from build123d import *

# Parameters (mm, degrees)
SKETCH1_R               = 114.3
BOSS_EXTRUDE1_DEPTH     = 762
SKETCH2_R               = 76.2
CUT_EXTRUDE1_DEPTH      = 94.996
CUT_EXTRUDE2_DEPTH      = 241.046
CUT_EXTRUDE2_DEPTH_BACK = 276.352
SKETCH6_R               = 150.368


with BuildPart() as part:
    # Sketch1 → Boss-Extrude1 (new body)
    with BuildSketch(Plane.XY):
        Circle(SKETCH1_R)
    extrude(amount=BOSS_EXTRUDE1_DEPTH)

    # Sketch2 → Cut-Extrude1 (cut)
    with BuildSketch(Plane.XY.offset(762)):
        Circle(SKETCH2_R)
    extrude(amount=-CUT_EXTRUDE1_DEPTH, mode=Mode.SUBTRACT)

    # Sketch6 → Cut-Extrude2 (cut, two sides: drawn at the far end of the back side and taken through both)
    with BuildSketch(Plane(origin=(0, 0, 0), x_dir=(1, 0, 0), z_dir=(0, 1, 0)).offset(-CUT_EXTRUDE2_DEPTH_BACK)):
        Circle(SKETCH6_R)
    extrude(amount=CUT_EXTRUDE2_DEPTH + CUT_EXTRUDE2_DEPTH_BACK, mode=Mode.SUBTRACT)


solid = part.part
Part model, mm, in its own coordinate system. A direction names the side the tool comes from. Give positions to 0.01 mm unless a question says otherwise; leave off trailing zeros. Loops run counter-clockwise (first coordinate to the right, second up) from the corner with the lowest first, then second, coordinate; pieces in that order, holes last. Notation, with made-up numbers: M -14,-38.75 L 6,-38.75 A11 ccw 6,-19.75 Z; hole C -35.75,89 d1. An arc over 180 degrees is marked long. Put each result on its own line as item: value. Start each with the question number.
1) Saw through at A-A (y = 0). List the corners of the cut face in (x, z), then the cut area to 3 significant figures.
2) Pull direction Y, two halves, no side cores. Call faces 1 (the flat face through (-1, 1, 667.004)), 2 (the cylindrical face through (-114.19, 5.03, 425.2)), 3 (the flat face through (24, -75, 762)): +Y half, -Y half, draft (parallel to the pull), parting line (faces both ways), or undercut.
3) Saw through at B-B (x = 0). List the corners of the cut face in (y, z).
4) Saw through at D-D (x = -93.5). List the corners of the cut face in (y, z), then the cut area to 3 significant figures.
5) Probe probe 1 along Y at (x, z) = (0, 693); probe 2 along Z at (x, y) = (0.5, 20.5); probe 3 along X at (y, z) = (-42, 705.5). List the from-to ranges inside material, lowest first.
6) Saw through at C-C (z = 181). List the corners of the cut face in (x, y), then the cut area to 3 significant figures.
7) Flat gauge pins, fed straight in: pin 1 (12 mm diameter, centred on y = -27, z = 185.5, fed in from +X); pin 2 (4 mm diameter, centred on x = -52.5, z = 174.5, fed in from -Y); pin 3 (5 mm diameter, centred on x = -75.5, z = 461, fed in from +Y). Where does each tip first touch, or does it go through?
8) 3-axis set-ups, long thin cutter, end or side, ignore diameter. For faces 4 (the cylindrical face through (-60.47, -46.367, 715.167)), 5 (the cylindrical face through (-1.818, -1.6, 150.357)): which of +Z, -Z, +X, -X, +Y, -Y reach the whole face in a straight line?
Numbers:
1. outline: M -114.3,97.7 A150.37 cw 114.3,97.7 L 114.3,762 L 76.2,762 L 76.2,667 L -76.2,667 L -76.2,762 L -114.3,762 Z
1. area: 129,000 mm^2
2. face 1: undercut
2. face 2: parting line
2. face 3: draft
3. outline: M -114.3,150.37 L 114.3,150.37 L 114.3,762 L 76.2,762 L 76.2,667 L -76.2,667 L -76.2,762 L -114.3,762 Z
4. outline: M -65.74,117.76 L 65.74,117.76 L 65.74,762 L -65.74,762 Z
4. area: 84,700 mm^2
5. probe 1: -114.3 to -76.2, 76.2 to 114.3
5. probe 2: 150.37 to 667
5. probe 3: -106.3 to -63.58, 63.58 to 106.3
6. outline: C 0,0 d228.6
6. area: 41,000 mm^2
7. pin 1: x = 112.35
7. pin 2: y = -102.54
7. pin 3: y = 87.95
8. face 4: +Z
8. face 5: -Z, +Y, -Y
